Verification items for the finished model (mm, model axes). A direction names the side the tool comes from. Round coordinates to 2 decimals unless told otherwise and drop trailing zeros. Write each loop counter-clockwise with the first axis right and the second up, starting at its lowest first coordinate (ties: lowest second). Pieces come first, ordered by that corner, then holes. Notation, with made-up numbers: (51, -25.75) - (97, -25.75) arc R26 cw to (97, -6.75) - close; hole circle Ø1 at (13.25, 43.5). An arc over 180 degrees is marked (long way). Answer as a JSON object with one key per item and string values.
```python
from build123d import *

# Parameters (mm, degrees)
BOSS_EXTRUDE1_DEPTH = 1.6
FILLET1_R           = 3
FILLET2_R           = 3
SKETCH3_R           = 7.6
CUT_EXTRUDE1_DEPTH  = 10
SCALE1_SCALE        = 1.15


with BuildPart() as part:
    # Sketch1 → Boss-Extrude1 (new body)
    with BuildSketch(Plane(origin=(0, 0, 0), x_dir=(1, 0, 0), z_dir=(0, 1, 0))):
        Polygon((-32.670459977, 56.192891409), (-64.999701461, -0.197002589), (-32.329241484, -56.389893998), (32.670459977, -56.192891409), (64.999701461, 0.197002589), (32.329241484, 56.389893998), align=None)
        with BuildLine():
            Line((-31.193440085, 47.277250649), (-56.559443422, 3.032901767))
            Line((-56.559443422, 3.032901767), (-15.685493875, 3.156783473))
            ThreePointArc((-15.685493875, 3.156783473), (-13.880589292, 7.957967134), (-10.649180608, 11.941312842))
            Line((-10.649180608, 11.941312842), (-31.193440085, 47.277250649))
        make_face(mode=Mode.SUBTRACT)
        with BuildLine():
            Line((-56.540020126, -3.375686221), (-30.906291689, -47.465463944))
            Line((-30.906291689, -47.465463944), (-10.576601619, -12.00564443))
            ThreePointArc((-10.576601619, -12.00564443), (-13.832096347, -8.041959379), (-15.666070579, -3.251804515))
            Line((-15.666070579, -3.251804515), (-56.540020126, -3.375686221))
        make_face(mode=Mode.SUBTRACT)
        with BuildLine():
            Line((-25.346580041, -50.65293687), (25.653151733, -50.498365711))
            Line((25.653151733, -50.498365711), (5.108892256, -15.162427903))
            ThreePointArc((5.108892256, -15.162427903), (0.048492945, -15.999926513), (-5.016889971, -15.193117357))
            Line((-5.016889971, -15.193117357), (-25.346580041, -50.65293687))
        make_face(mode=Mode.SUBTRACT)
        with BuildLine():
            Line((31.193440085, -47.277250649), (56.559443422, -3.032901767))
            Line((56.559443422, -3.032901767), (15.685493875, -3.156783473))
            ThreePointArc((15.685493875, -3.156783473), (13.880589292, -7.957967134), (10.649180608, -11.941312842))
            Line((10.649180608, -11.941312842), (31.193440085, -47.277250649))
        make_face(mode=Mode.SUBTRACT)
        with BuildLine():
            Line((56.540020126, 3.375686221), (30.906291689, 47.465463944))
            Line((30.906291689, 47.465463944), (10.576601619, 12.00564443))
            ThreePointArc((10.576601619, 12.00564443), (13.832096347, 8.041959379), (15.666070579, 3.251804515))
            Line((15.666070579, 3.251804515), (56.540020126, 3.375686221))
        make_face(mode=Mode.SUBTRACT)
        with BuildLine():
            Line((25.346580041, 50.65293687), (-25.653151733, 50.498365711))
            Line((-25.653151733, 50.498365711), (-5.108892256, 15.162427903))
            ThreePointArc((-5.108892256, 15.162427903), (-0.048492945, 15.999926513), (5.016889971, 15.193117357))
            Line((5.016889971, 15.193117357), (25.346580041, 50.65293687))
        make_face(mode=Mode.SUBTRACT)
        Polygon((28.764451985, 52.408726504), (31.157091964, 51.352131998), (32.90133947, 53.301162184), (31.586703733, 55.562323589), (29.029966659, 55.010768007), align=None, mode=Mode.SUBTRACT)
        Polygon((-31.00506254, 51.115109397), (-28.893704867, 52.658899148), (-29.709490768, 55.143976891), (-32.325031855, 55.136049649), (-33.125739246, 52.646072601), align=None, mode=Mode.SUBTRACT)
        Polygon((59.769514525, 1.293617108), (60.050796831, -1.30676715), (62.610830237, -1.842814707), (63.911735588, 0.42627394), (62.155705905, 2.364695405), align=None, mode=Mode.SUBTRACT)
        Polygon((31.00506254, -51.115109397), (28.893704867, -52.658899148), (29.709490768, -55.143976891), (32.325031855, -55.136049649), (33.125739246, -52.646072601), align=None, mode=Mode.SUBTRACT)
        Polygon((-28.764451985, -52.408726504), (-31.157091964, -51.352131998), (-32.90133947, -53.301162184), (-31.586703733, -55.562323589), (-29.029966659, -55.010768007), align=None, mode=Mode.SUBTRACT)
        Polygon((-59.769514525, -1.293617108), (-60.050796831, 1.30676715), (-62.610830237, 1.842814707), (-63.911735588, -0.42627394), (-62.155705905, -2.364695405), align=None, mode=Mode.SUBTRACT)
    extrude(amount=BOSS_EXTRUDE1_DEPTH)

    # Fillet1
    fillet1_edges = [part.edges().sort_by_distance(p)[0] for p in [
        (32.329241484, 0.8, -56.389893998),
        (64.999701461, 0.8, -0.197002589),
        (32.670459977, 0.8, 56.192891409),
        (-32.329241484, 0.8, 56.389893998),
        (-64.999701461, 0.8, 0.197002589),
        (-32.670459977, 0.8, -56.192891409),
    ]]
    fillet(fillet1_edges, radius=FILLET1_R)

    # Fillet2
    fillet2_edges = [part.edges().sort_by_distance(p)[0] for p in [
        (-25.653151733, 0.8, -50.498365711),
        (-5.108892256, 0.8, -15.162427903),
        (5.016889971, 0.8, -15.193117357),
        (25.346580041, 0.8, -50.65293687),
        (30.906291689, 0.8, -47.465463944),
        (10.576601619, 0.8, -12.00564443),
        (15.666070579, 0.8, -3.251804515),
        (56.540020126, 0.8, -3.375686221),
        (56.559443422, 0.8, 3.032901767),
        (15.685493875, 0.8, 3.156783473),
        (10.649180608, 0.8, 11.941312842),
        (31.193440085, 0.8, 47.277250649),
        (25.653151733, 0.8, 50.498365711),
        (5.108892256, 0.8, 15.162427903),
        (-5.016889971, 0.8, 15.193117357),
        (-25.346580041, 0.8, 50.65293687),
        (-30.906291689, 0.8, 47.465463944),
        (-10.576601619, 0.8, 12.00564443),
        (-15.666070579, 0.8, 3.251804515),
        (-56.540020126, 0.8, 3.375686221),
        (-10.649180608, 0.8, -11.941312842),
        (-31.193440085, 0.8, -47.277250649),
        (-56.559443422, 0.8, -3.032901767),
        (-15.685493875, 0.8, -3.156783473),
    ]]
    fillet(fillet2_edges, radius=FILLET2_R)

    # Sketch3 → Cut-Extrude1 (cut)
    with BuildSketch(Plane(origin=(0, 3.6, 0), x_dir=(1, 0, 0), z_dir=(0, 1, 0))):
        with Locations(Location((0, 0, 0), (0, 0, 270))):
            Circle(SKETCH3_R)
    extrude(amount=-CUT_EXTRUDE1_DEPTH, mode=Mode.SUBTRACT)


with BuildPart() as part_1:
    # Scale1: scaled about (0, 0.8, 0)
    add(part.part.scale(SCALE1_SCALE).moved(Location((0, -0.12, 0))))


solid = part_1.part
```
Q1. Section check C-C, the plane x = 55. Record the cut outline in (y, z).
Geometry check:
{"outline": "(-0.12, -34.2) - (1.72, -34.2) - (1.72, -21.12) - (-0.12, -21.12) - close; (-0.12, -3.85) - (1.72, -3.85) - (1.72, 3.52) - (-0.12, 3.52) - close; (-0.12, 21.01) - (1.72, 21.01) - (1.72, 34.22) - (-0.12, 34.22) - close"}
Q2. Material ranges on line 1 along X through (y, z) = (1.45, -27.5); line 2 along X through (y, z) = (0.3, -45); line 3 along Z through (x, y) = (20, 0.2), recorded low to high. Write a range as [from, to].
Geometry check:
{"line 1": "x = [-58.85, -51.28], [-20.25, -11.73], [11.52, 20.01], [51.29, 58.89]", "line 2": "x = [-48.82, -41.24], [-30.43, -21.9], [21.55, 30.05], [41.12, 48.72]", "line 3": "z = [-64.8, -58.22], [-42.29, -27.48], [-3.81, 3.69], [27.07, 41.73], [58.1, 64.68]"}
Q3. Section check D-D, the plane y = 1.2. State how many separate pieces and enclosed holes the cut face has, then the cut area to 3 significant figures.
Geometry check:
{"separate pieces": "1", "enclosed holes": "13", "area": "5,750 mm2"}
Q4. Section check B-B, the plane z = 44. Record the cut outline in (x, y).
Geometry check:
{"outline": "(-49.3, -0.12) - (-41.7, -0.12) - (-41.7, 1.72) - (-49.3, 1.72) - close; (-29.47, -0.12) - (-20.98, -0.12) - (-20.98, 1.72) - (-29.47, 1.72) - close; (21.32, -0.12) - (29.84, -0.12) - (29.84, 1.72) - (21.32, 1.72) - close; (41.82, -0.12) - (49.39, -0.12) - (49.39, 1.72) - (41.82, 1.72) - close"}
Q5. Release check for a two-part mould opening along Z. For faces 1 (the flat face through (-56.213, 0.787, 32.109)), 2 (the cylindrical face through (15.882, 0.787, -9.291)), 3 (the flat face through (-55.914, 0.787, -32.627)) record: released by +Z, released by -Z, zero draft, split by the parting line, or undercut.
Geometry check:
{"face 1": "released by +Z", "face 2": "undercut", "face 3": "released by -Z"}
Q6. Set-up check for faces 4 (the flat face through (5, -0.12, 9)), 5 (the flat face through (50.3, 0.8, 29.2)): record each of +Z, -Z, +X, -X, +Y, -Y from which the full face is reachable in a straight line by a thin tool's end or side.
Geometry check:
{"face 4": "+Z, -Z, +X, -X, -Y", "face 5": "+Y, -Y"}
Q7. Section check A-A, the plane x = 0. Record the cut outline in (y, z).
Geometry check:
{"outline": "(-0.12, -64.74) - (1.72, -64.74) - (1.72, -58.16) - (-0.12, -58.16) - close; (-0.12, -18.4) - (1.72, -18.4) - (1.72, -8.74) - (-0.12, -8.74) - close; (-0.12, 8.74) - (1.72, 8.74) - (1.72, 18.4) - (-0.12, 18.4) - close; (-0.12, 58.16) - (1.72, 58.16) - (1.72, 64.74) - (-0.12, 64.74) - close"}
